Geometry check sheet. Reference: the model listing, model coordinates, mm. A direction names the side the tool comes from. Coordinates: 2 decimals unless noted, no trailing zeros. Order: outer loops, then holes, each group sorted by start corner. A loop starts at its lowest first (then second) coordinate and runs counter-clockwise, first axis right, second up. Notation, with made-up numbers: (64.25, -21.5) - (94.25, -21.5) arc R25 cw to (94.25, 11.5) - close; hole circle Ø10 at (33, 29.25). An arc over 180 degrees is marked (long way). One line per item, written item: value. Start each with the question number.
```python
from build123d import *

# Parameters (mm, degrees)
SKETCH1_R                   = 13.5
BASE_SIZE_DEPTH             = 5
MOUNTING_HOLES_REACH        = 21.736
SKETCH2_R                   = 1
SKETCH3_R                   = 12.5
ROTOR_POCKET_DEPTH          = 2.5
ROTOR_POCKET_DRAFT          = -15
OUTSIDE_CHAMFER_SIZE        = 5
OUTSIDE_CHAMFER_SIZE_2      = 1.339745962
BOTTOM_POCKETS_TOP_DEPTH    = 1.55
BOTTOM_POCKETS_BOTTOM_DEPTH = 2.15
BOTTOM_POCKETS_FILLET_R     = 5
CUT_EXTRUDE5_REACH          = 21.736
SKETCH6_R                   = 4
CHAMFER2_SIZE               = 1.4
SKETCH7_R                   = 4.8
SKETCH7_R_2                 = 4
BEARING_BOTTOM_DEPTH        = 3
SKETCH8_R                   = 4.8
SKETCH8_R_2                 = 3.2
BEARING_SEPARATOR_DEPTH     = 1
SKETCH9_R                   = 4.8
SKETCH9_R_2                 = 4
BEARING_TOP_DEPTH           = 4
CUT_EXTRUDE6_DEPTH          = 2.05


with BuildPart() as part:
    # Sketch1 → Base size (new body)
    with BuildSketch(Plane(origin=(0, 0, 0), x_dir=(1, 0, 0), z_dir=(0, 1, 0))):
        with Locations(Location((0, 0, 0), (0, 0, 270))):
            Circle(SKETCH1_R)
    extrude(amount=BASE_SIZE_DEPTH)

    # Sketch2 → Mounting holes (cut, up to next)
    with BuildSketch(Plane(origin=(0, 5, 0), x_dir=(1, 0, 0), z_dir=(0, 1, 0)), mode=Mode.PRIVATE) as mounting_holes_sk1:
        with Locations(Location((5.656854249, 5.656854249, 0), (0, 0, 270))):
            Circle(SKETCH2_R)
    mounting_holes_tool1 = extrude(mounting_holes_sk1.sketch, amount=-MOUNTING_HOLES_REACH, mode=Mode.PRIVATE) & part.part
    # Sketch2 → Mounting holes (cut, up to next)
    with BuildSketch(Plane(origin=(0, 5, 0), x_dir=(1, 0, 0), z_dir=(0, 1, 0)), mode=Mode.PRIVATE) as mounting_holes_sk2:
        with Locations(Location((-5.656854249, -5.656854249, 0), (0, 0, 270))):
            Circle(SKETCH2_R)
    mounting_holes_tool2 = extrude(mounting_holes_sk2.sketch, amount=-MOUNTING_HOLES_REACH, mode=Mode.PRIVATE) & part.part
    # Sketch2 → Mounting holes (cut, up to next)
    with BuildSketch(Plane(origin=(0, 5, 0), x_dir=(1, 0, 0), z_dir=(0, 1, 0)), mode=Mode.PRIVATE) as mounting_holes_sk3:
        with Locations(Location((5.656854249, -5.656854249, 0), (0, 0, 270))):
            Circle(SKETCH2_R)
    mounting_holes_tool3 = extrude(mounting_holes_sk3.sketch, amount=-MOUNTING_HOLES_REACH, mode=Mode.PRIVATE) & part.part
    # Sketch2 → Mounting holes (cut, up to next)
    with BuildSketch(Plane(origin=(0, 5, 0), x_dir=(1, 0, 0), z_dir=(0, 1, 0)), mode=Mode.PRIVATE) as mounting_holes_sk4:
        with Locations(Location((-5.656854249, 5.656854249, 0), (0, 0, 270))):
            Circle(SKETCH2_R)
    mounting_holes_tool4 = extrude(mounting_holes_sk4.sketch, amount=-MOUNTING_HOLES_REACH, mode=Mode.PRIVATE) & part.part
    add(mounting_holes_tool1.solids().sort_by_distance((5.656854, 5, -5.656854))[0], mode=Mode.SUBTRACT)
    add(mounting_holes_tool2.solids().sort_by_distance((-5.656854, 5, 5.656854))[0], mode=Mode.SUBTRACT)
    add(mounting_holes_tool3.solids().sort_by_distance((5.656854, 5, 5.656854))[0], mode=Mode.SUBTRACT)
    add(mounting_holes_tool4.solids().sort_by_distance((-5.656854, 5, -5.656854))[0], mode=Mode.SUBTRACT)


with BuildPart() as rotor_pocket_tool:
    # Sketch3 → Rotor pocket (with draft: the straight prism first)
    with BuildSketch(Plane.XZ):
        Circle(SKETCH3_R)
    extrude(amount=-ROTOR_POCKET_DEPTH)
    # Rotor pocket: the draft: its side faces are tilted about the plane it starts from
    rotor_pocket_sides = [rotor_pocket_tool.faces().sort_by_distance(p)[0] for p in [
        (-12.5, 1.25, 0),
    ]]
    draft(rotor_pocket_sides, Plane.XZ, ROTOR_POCKET_DRAFT)


with BuildPart() as part_1:
    add(part.part)

    # Rotor pocket: cut by rotor_pocket_tool
    add(rotor_pocket_tool.part, mode=Mode.SUBTRACT)

    # Outside chamfer
    # the kernel refuses this chamfer: 5, 1.339745962 mm, written as the material it takes off along each edge
    with BuildSketch(Plane(origin=(0, 5, 0), x_dir=(0, 0, 1), z_dir=(-1, 0, 0))) as outside_chamfer_piece_1:
        Polygon((13.5, -OUTSIDE_CHAMFER_SIZE), (13.5 - OUTSIDE_CHAMFER_SIZE_2, 0), (13.5, 0), align=None)
    revolve(axis=Axis((0, 5, 0), (0, 1, 0)), mode=Mode.SUBTRACT)

    # Sketch4 → Bottom pockets top (cut)
    with BuildSketch(Plane(origin=(0, 5, 0), x_dir=(1, 0, 0), z_dir=(0, 1, 0))):
        with BuildLine():
            Line((-3.889087297, 0), (-10.320380271, 6.431292975))
            ThreePointArc((-10.320380271, 6.431292975), (-12.160254038, 0), (-10.320380271, -6.431292975))
            Line((-10.320380271, -6.431292975), (-3.889087297, 0))
        make_face()
        with BuildLine():
            Line((-10.320380271, 6.431292975), (-10.543141739, 6.654054443))
            Line((-10.543141739, 6.654054443), (-11.29033147, 7.401244173))
            ThreePointArc((-11.29033147, 7.401244173), (-13.5, 0), (-11.29033147, -7.401244173))
            Line((-11.29033147, -7.401244173), (-10.543141739, -6.654054443))
            Line((-10.543141739, -6.654054443), (-10.320380271, -6.431292975))
            ThreePointArc((-10.320380271, -6.431292975), (-12.160254038, 0), (-10.320380271, 6.431292975))
        make_face()
        with BuildLine():
            ThreePointArc((6.431292975, 10.320380271), (0, 12.160254038), (-6.431292975, 10.320380271))
            Line((-6.431292975, 10.320380271), (0, 3.889087297))
            Line((0, 3.889087297), (6.431292975, 10.320380271))
        make_face()
        with BuildLine():
            Line((-6.654054443, 10.543141739), (-6.431292975, 10.320380271))
            ThreePointArc((-6.431292975, 10.320380271), (0, 12.160254038), (6.431292975, 10.320380271))
            Line((6.431292975, 10.320380271), (6.654054443, 10.543141739))
            Line((6.654054443, 10.543141739), (7.401244173, 11.29033147))
            ThreePointArc((7.401244173, 11.29033147), (0, 13.5), (-7.401244173, 11.29033147))
            Line((-7.401244173, 11.29033147), (-6.654054443, 10.543141739))
        make_face()
        with BuildLine():
            Line((10.320380271, 6.431292975), (3.889087297, 0))
            Line((3.889087297, 0), (10.320380271, -6.431292975))
            ThreePointArc((10.320380271, -6.431292975), (11.691240827, -3.344647396), (12.160254038, 0))
            ThreePointArc((12.160254038, 0), (11.691240827, 3.344647396), (10.320380271, 6.431292975))
        make_face()
        with BuildLine():
            Line((10.543141739, 6.654054443), (10.320380271, 6.431292975))
            ThreePointArc((10.320380271, 6.431292975), (11.691240827, 3.344647396), (12.160254038, 0))
            ThreePointArc((12.160254038, 0), (11.691240827, -3.344647396), (10.320380271, -6.431292975))
            Line((10.320380271, -6.431292975), (10.543141739, -6.654054443))
            Line((10.543141739, -6.654054443), (11.29033147, -7.401244173))
            ThreePointArc((11.29033147, -7.401244173), (12.935792879, -3.862028299), (13.5, 0))
            ThreePointArc((13.5, 0), (12.935792879, 3.862028299), (11.29033147, 7.401244173))
            Line((11.29033147, 7.401244173), (10.543141739, 6.654054443))
        make_face()
        with BuildLine():
            ThreePointArc((6.431292975, -10.320380271), (0, -12.160254038), (-6.431292975, -10.320380271))
            Line((-6.431292975, -10.320380271), (-6.654054443, -10.543141739))
            Line((-6.654054443, -10.543141739), (-7.401244173, -11.29033147))
            ThreePointArc((-7.401244173, -11.29033147), (0, -13.5), (7.401244173, -11.29033147))
            Line((7.401244173, -11.29033147), (6.654054443, -10.543141739))
            Line((6.654054443, -10.543141739), (6.431292975, -10.320380271))
        make_face()
        with BuildLine():
            Line((6.431292975, -10.320380271), (0, -3.889087297))
            Line((0, -3.889087297), (-6.431292975, -10.320380271))
            ThreePointArc((-6.431292975, -10.320380271), (0, -12.160254038), (6.431292975, -10.320380271))
        make_face()
    extrude(amount=-BOTTOM_POCKETS_TOP_DEPTH, mode=Mode.SUBTRACT)

    # Sketch5 → Bottom pockets bottom (cut)
    with BuildSketch(Plane(origin=(0, 3.45, 0), x_dir=(1, 0, 0), z_dir=(0, 1, 0))):
        with BuildLine():
            ThreePointArc((-10.621599421, 6.732512125), (-12.575575286, 0), (-10.621599421, -6.732512125))
            Line((-10.621599421, -6.732512125), (-3.889087297, 0))
            Line((-3.889087297, 0), (-10.621599421, 6.732512125))
        make_face()
        with BuildLine():
            Line((-10.621599421, 6.732512125), (-11.29033147, 7.401244173))
            ThreePointArc((-11.29033147, 7.401244173), (-13.5, 0), (-11.29033147, -7.401244173))
            Line((-11.29033147, -7.401244173), (-10.621599421, -6.732512125))
            ThreePointArc((-10.621599421, -6.732512125), (-12.575575286, 0), (-10.621599421, 6.732512125))
        make_face()
        with BuildLine():
            ThreePointArc((7.401244173, 11.29033147), (0, 13.5), (-7.401244173, 11.29033147))
            Line((-7.401244173, 11.29033147), (0, 3.889087297))
            Line((0, 3.889087297), (7.401244173, 11.29033147))
        make_face()
        with BuildLine():
            Line((11.29033147, 7.401244173), (3.889087297, 0))
            Line((3.889087297, 0), (11.29033147, -7.401244173))
            ThreePointArc((11.29033147, -7.401244173), (12.935792879, -3.862028299), (13.5, 0))
            ThreePointArc((13.5, 0), (12.935792879, 3.862028299), (11.29033147, 7.401244173))
        make_face()
    extrude(amount=-BOTTOM_POCKETS_BOTTOM_DEPTH, mode=Mode.SUBTRACT)

    # Bottom pockets fillet
    bottom_pockets_fillet_edges = [part_1.edges().sort_by_distance(p)[0] for p in [
        (-3.889087297, 3.75, 0),
        (3.889087297, 3.75, 0),
        (0, 4.225, 3.889087297),
        (0, 3.75, -3.889087297),
    ]]
    fillet(bottom_pockets_fillet_edges, radius=BOTTOM_POCKETS_FILLET_R)

    # Sketch6 → Cut-Extrude5 (cut, up to next)
    with BuildSketch(Plane(origin=(0, 5, 0), x_dir=(1, 0, 0), z_dir=(0, 1, 0)), mode=Mode.PRIVATE) as cut_extrude5_sk1:
        with Locations(Location((0, 0, 0), (0, 0, 270))):
            Circle(SKETCH6_R)
    cut_extrude5_tool1 = extrude(cut_extrude5_sk1.sketch, amount=-CUT_EXTRUDE5_REACH, mode=Mode.PRIVATE) & part_1.part
    add(cut_extrude5_tool1.solids().sort_by_distance((0, 5, 0))[0], mode=Mode.SUBTRACT)

    # Chamfer2
    chamfer2_edges = [part_1.edges().sort_by_distance(p)[0] for p in [
        (0, 5, -4),
    ]]
    chamfer(chamfer2_edges, length=CHAMFER2_SIZE)

    # Sketch7 → Bearing bottom (add)
    with BuildSketch(Plane.XZ.offset(-2.5)):
        with Locations(Location((0, 0, 0), (0, 0, 270))):
            Circle(SKETCH7_R)
        with Locations(Location((0, 0, 0), (0, 0, 90))):
            Circle(SKETCH7_R_2, mode=Mode.SUBTRACT)
    extrude(amount=BEARING_BOTTOM_DEPTH)

    # Sketch8 → Bearing separator (add)
    with BuildSketch(Plane.XZ.offset(0.5)):
        with Locations(Location((0, 0, 0), (0, 0, 270))):
            Circle(SKETCH8_R)
        with Locations(Location((0, 0, 0), (0, 0, 270))):
            Circle(SKETCH8_R_2, mode=Mode.SUBTRACT)
    extrude(amount=BEARING_SEPARATOR_DEPTH)

    # Sketch9 → Bearing top (add)
    with BuildSketch(Plane.XZ.offset(1.5)):
        with Locations(Location((0, 0, 0), (0, 0, 270))):
            Circle(SKETCH9_R)
        with Locations(Location((0, 0, 0), (0, 0, 90))):
            Circle(SKETCH9_R_2, mode=Mode.SUBTRACT)
    extrude(amount=BEARING_TOP_DEPTH)

    # Sketch10 → Cut-Extrude6 (cut)
    with BuildSketch(Plane(origin=(0, 3.45, 0), x_dir=(1, 0, 0), z_dir=(0, 1, 0))):
        with BuildLine():
            ThreePointArc((-1.167513596, -10.937865971), (-1.779893821, -10.094279468), (-2.643866576, -10.677545108))
            Line((-2.643866576, -10.677545108), (-3.078810633, -13.144235432))
            ThreePointArc((-3.078810633, -13.144235432), (-2.344250399, -13.294904666), (-1.602457654, -13.404556295))
            Line((-1.602457654, -13.404556295), (-1.167513596, -10.937865971))
        make_face()
        with BuildLine():
            ThreePointArc((2.643866576, -10.677545108), (1.779893821, -10.094279468), (1.167513596, -10.937865971))
            Line((1.167513596, -10.937865971), (1.602457654, -13.404556295))
            ThreePointArc((1.602457654, -13.404556295), (2.344250399, -13.294904666), (3.078810633, -13.144235432))
            Line((3.078810633, -13.144235432), (2.643866576, -10.677545108))
        make_face()
        with BuildLine():
            Line((-0.75, -11), (-0.75, -13.479150567))
            ThreePointArc((-0.75, -13.479150567), (0, -13.5), (0.75, -13.479150567))
            Line((0.75, -13.479150567), (0.75, -11))
            ThreePointArc((0.75, -11), (0, -10.25), (-0.75, -11))
        make_face()
    extrude(amount=-CUT_EXTRUDE6_DEPTH, mode=Mode.SUBTRACT)


solid = part_1.part
```
Q1. Release check for a two-part mould opening along X. For faces 5 (the flat face through (-12.4, 1.3, -0.1)), 6 (the cylindrical face through (-1.947, -0.993, 2.539)), 7 (the conical face through (8.26, 4.76, -9.01)) record: released by +X, released by -X, zero draft, split by the parting line, or undercut.
Q2. Material ranges on probe 1 along X at (y, z) = (-2.5, -0.25); probe 2 along X at (y, z) = (2.75, 5.5); probe 3 along X at (y, z) = (1.25, -1.25), recorded low to high.
Q3. Cross-section at A-A, the plane z = 0. Count the separate pieces of the cut face and the enclosed holes in it, and give its area (3 significant figures).
Q4. Cross-section at B-B, the plane y = -2.5. Enter the section's corners in (x, z).
Q5. Gauge pin test, flat ends, axial feed: P1, Ø0.9, axis at x = -12.5, z = -2, coming from the +Y side; P2, Ø1, axis at y = 3, z = -10.5, coming from the +X side; P3, Ø6.5, axis at x = 0, z = 0, coming from the +Y side; P4, Ø4, axis at x = 1.5, z = 3.5, coming from the -Y side. Record the tip position at first contact, or that the pin passes through.
Q6. Set-up check for faces 1 (the flat face through (3, -0.5, 2)), 2 (the flat face through (-2.826, 2.667, 11.711)), 3 (the flat face through (-0.1, 1.3, -12.4)), 4 (the cylindrical face through (3.905, -3.472, -0.867)): record each of +Z, -Z, +X, -X, +Y, -Y from which the full face is reachable in a straight line by a thin tool's end or side.
Check result:
1. face 5: zero draft
1. face 6: undercut
1. face 7: split by the parting line
2. probe 1: x = -4.79 to -3.99, 3.99 to 4.79
2. probe 2: x = -9.39 to -6.64, -4.67 to 4.67, 6.64 to 9.39
2. probe 3: x = -13.11 to -12.1, -4.63 to -3.8, 3.8 to 4.63, 12.1 to 13.11
3. separate pieces: 4
3. enclosed holes: 0
3. area: 24.8 mm2
4. outline: circle Ø9.6 at (0, 0); hole circle Ø8 at (0, 0)
5. P1: stops at y = 1.3
5. P2: stops at x = 7.86
5. P3: stops at y = -0.5
5. P4: stops at y = -5.5
6. face 1: +Y
6. face 2: +Z, +Y
6. face 3: -Z, +Y
6. face 4: -Y
